from build123d import *

# Parameters (mm, degrees)
SKETCH_2_R      = 0.4
EXTRUDE_1_DEPTH = 6.5


with BuildPart() as part:
    # 草图1 → 旋转1 (revolve)
    with BuildSketch(Plane(origin=(0, 0, 0), x_dir=(1, 0, 0), z_dir=(0, 1, 0)), mode=Mode.PRIVATE) as revolve_1_sk:
        with BuildLine():
            Line((0, 8), (0, 0))
            Line((0, 0), (8.5, 0))
            Line((8.5, 0), (8.5, 9))
            ThreePointArc((8.5, 9), (8.207106781, 9.707106781), (7.5, 10))
            Line((7.5, 10), (4.55, 10))
            ThreePointArc((4.55, 10), (4.337867966, 9.912132034), (4.25, 9.7))
            Line((4.25, 9.7), (4.25, 8.3))
            ThreePointArc((4.25, 8.3), (4.162132034, 8.087867966), (3.95, 8))
            Line((3.95, 8), (0, 8))
        make_face()
    revolve(revolve_1_sk.sketch.rotate(Axis((0, 0, -9.831715268), (0, 0, 1)), 180), axis=Axis((0, 0, -9.831715268), (0, 0, 1)))

    # 草图2 → 凸台-拉伸1 (add)
    with BuildSketch(Plane.XY):
        with Locations(Location((-4.75, 0, 0), (0, 0, 180))):
            Circle(SKETCH_2_R)
        with Locations(Location((-3.358757211, 3.358757211, 0), (0, 0, 180))):
            Circle(SKETCH_2_R)
        with Locations(Location((3.358757211, 3.358757211, 0), (0, 0, 180))):
            Circle(SKETCH_2_R)
        with Locations(Location((4.75, 0, 0), (0, 0, 180))):
            Circle(SKETCH_2_R)
        with Locations(Location((3.358757211, -3.358757211, 0), (0, 0, 180))):
            Circle(SKETCH_2_R)
        with Locations(Location((-3.358757211, -3.358757211, 0), (0, 0, 180))):
            Circle(SKETCH_2_R)
    extrude(amount=EXTRUDE_1_DEPTH)


solid = part.part
Can you work these out from the model? Positions are in its coordinate system, mm. A direction names the side the tool comes from. Give positions to 0.01 mm unless a question says otherwise; leave off trailing zeros. Order: outer loops, then holes, each group sorted by start corner. A loop starts at its lowest first (then second) coordinate and runs counter-clockwise, first axis right, second up. Notation, with made-up numbers: M 4,43 L 26,43 A25 cw 26,73 Z; hole C 37,54 d7. An arc over 180 degrees is marked long. Use a Markdown table: item, result. Add a question column.
Item 1: Suppose I cut it at B-B (x = 0). List the corners of the cut face in (y, z) for me, then the cut area to 3 significant figures.
Item 2: If I drill on L1, parallel to Y at x = 0, z = -8.7; L2, parallel to Z at x = -3.5, y = 1; L3, parallel to Z at x = -3.5, y = -6, over which ranges is the centre line in solid material (lowest first)? Write a range as [from, to].
Item 3: Suppose I cut it at D-D (z = -3.75). List the corners of the cut face in (x, y) for me, then the cut area to 3 significant figures.
Item 4: For faces 1 (the cylindrical face through (1.107, -8.428, -4.563)), 2 (the cylindrical face through (-4.455, -0.27, 3.204)), which set-ups out of +Z, -Z, +X, -X, +Y, -Y let a thin tool reach every point of the face, with its end or its side?
Item 5: Will these pins go through, and if not, where does the flat tip stop? pin 1 (1 mm diameter, centred on x = 6, y = 6.5, fed in from -Z); pin 2 (5 mm diameter, centred on x = 0, y = 0, fed in from +Z); pin 3 (1 mm diameter, centred on x = 3, z = -4, fed in from -Y).
Item 6: Suppose I cut it at C-C (z = 4.5). List the corners of the cut face in (x, y) for me, then the cut area to 3 significant figures.
Item 7: We'd pull the mould along Y, two halves only. Please class faces 3 (the flat face through (0, 5, -10)), 4 (the cylindrical face through (5.045, -0.27, 3.204)), 5 (the flat face through (0, 0, -8)), 6 (the cylindrical face through (0.553, -4.214, -8.99)): +Y half, -Y half, draft (parallel to the pull), parting line (faces both ways), or undercut.
Item 8: Suppose I cut it at A-A (y = 0). List the corners of the cut face in (x, z) for me.
Answer sheet:
| question | item | result |
|---|---|---|
| 1 | outline | M -8.5,-9 A1 ccw -7.5,-10 L -4.55,-10 A0.3 ccw -4.25,-9.7 L -4.25,-8.3 A0.3 cw -3.95,-8 L 3.95,-8 A0.3 cw 4.25,-8.3 L 4.25,-9.7 A0.3 ccw 4.55,-10 L 7.5,-10 A1 ccw 8.5,-9 L 8.5,0 L -8.5,0 Z |
| 1 | area | 153 mm² |
| 2 | L1 | y = [-8.5, -4.25], [4.25, 8.5] |
| 2 | L2 | z = [-8, 0] |
| 2 | L3 | z = [-10, 0] |
| 3 | outline | C 0,0 d17 |
| 3 | area | 227 mm² |
| 4 | face 1 | +Z, -Z |
| 4 | face 2 | +Z |
| 5 | pin 1 | stops at z = -9.53 |
| 5 | pin 2 | stops at z = 0 |
| 5 | pin 3 | stops at y = -8.12 |
| 6 | outline | C -4.75,0 d0.8; C -3.36,-3.36 d0.8; C -3.36,3.36 d0.8; C 3.36,-3.36 d0.8; C 3.36,3.36 d0.8; C 4.75,0 d0.8 |
| 6 | area | 3.02 mm² |
| 7 | face 3 | draft |
| 7 | face 4 | parting line |
| 7 | face 5 | undercut |
| 7 | face 6 | undercut |
| 8 | outline | M -8.5,-9 A1 ccw -7.5,-10 L -4.55,-10 A0.3 ccw -4.25,-9.7 L -4.25,-8.3 A0.3 cw -3.95,-8 L 3.95,-8 A0.3 cw 4.25,-8.3 L 4.25,-9.7 A0.3 ccw 4.55,-10 L 7.5,-10 A1 ccw 8.5,-9 L 8.5,0 L 5.15,0 L 5.15,6.5 L 4.35,6.5 L 4.35,0 L -4.35,0 L -4.35,6.5 L -5.15,6.5 L -5.15,0 L -8.5,0 Z |
